Geometry check sheet. Reference: the model listing, model coordinates, mm. A direction names the side the tool comes from. Round coordinates to 2 decimals unless told otherwise and drop trailing zeros. Order: outer loops, then holes, each group sorted by start corner. A loop starts at its lowest first (then second) coordinate and runs counter-clockwise, first axis right, second up.
```python
from build123d import *

# Parameters (mm, degrees)
SKETCH1_R           = 1.5
BOSS_EXTRUDE1_DEPTH = 3
SKETCH4_R           = 1.5
CUT_EXTRUDE2_DEPTH  = 7
SKETCH5_W           = 46.5
SKETCH5_H           = 2
CUT_EXTRUDE3_DEPTH  = 7
CUT_EXTRUDE4_DEPTH  = 7
CUT_EXTRUDE5_DEPTH  = 7
BOSS_EXTRUDE2_START = -6
SKETCH8_R           = 1.5
BOSS_EXTRUDE2_DEPTH = 6
SKETCH9_R           = 1.5
CUT_EXTRUDE6_DEPTH  = 6
SKETCH10_R          = 1.5
CUT_EXTRUDE7_DEPTH  = 6
SKETCH11_W          = 36.769244088
SKETCH11_H          = 16.925373541
CUT_EXTRUDE8_DEPTH  = 14
FILLET2_R           = 5
FILLET3_R           = 10
FILLET4_R           = 20
FILLET5_R           = 30
FILLET6_R           = 10


with BuildPart() as part:
    # Sketch1 → Boss-Extrude1 (new body)
    # profile 1 of 4: a face of its own
    with BuildSketch(Plane(origin=(0, 0, 0), x_dir=(1, 0, 0), z_dir=(0, 1, 0))):
        Polygon((5, 16.666723622), (5, 56.73), (-5, 56.73), (-5, 5.234024539), (5, 5.234024539), (31.5, 5.234024539), (41.5, 5.234024539), (41.5, 64.6), (31.5, 64.6), (31.5, 54.48), (31.5, 16.666723622), align=None)
        with Locations(Location((0, 10.18, 0), (0, 0, 270))):
            Circle(SKETCH1_R, mode=Mode.SUBTRACT)
        with Locations(Location((36.5, 11.18, 0), (0, 0, 270))):
            Circle(SKETCH1_R, mode=Mode.SUBTRACT)
        with Locations(Location((0, 51.73, 0), (0, 0, 270))):
            Circle(SKETCH1_R, mode=Mode.SUBTRACT)
        with Locations(Location((36.5, 49.6, 0), (0, 0, 270))):
            Circle(SKETCH1_R, mode=Mode.SUBTRACT)
        with Locations(Location((36.5, 59.6, 0), (0, 0, 270))):
            Circle(SKETCH1_R, mode=Mode.SUBTRACT)
    # profile 2 of 4: a face of its own
    with BuildSketch(Plane(origin=(0, 0, 0), x_dir=(1, 0, 0), z_dir=(0, 1, 0))):
        Polygon((-5, 56.73), (5, 56.73), (31.5, 54.48), (31.5, 64.6), align=None)
    # profile 3 of 4: a face of its own
    with BuildSketch(Plane(origin=(0, 0, 0), x_dir=(1, 0, 0), z_dir=(0, 1, 0))):
        Polygon((5, 16.666723622), (5, 56.73), (-5, 56.73), (-5, 5.234024539), (5, 5.234024539), (31.5, 5.234024539), (41.5, 5.234024539), (41.5, 64.6), (31.5, 64.6), (31.5, 54.48), (31.5, 16.666723622), align=None)
        with Locations(Location((0, 10.18, 0), (0, 0, 270))):
            Circle(SKETCH1_R, mode=Mode.SUBTRACT)
        with Locations(Location((36.5, 11.18, 0), (0, 0, 270))):
            Circle(SKETCH1_R, mode=Mode.SUBTRACT)
        with Locations(Location((0, 51.73, 0), (0, 0, 270))):
            Circle(SKETCH1_R, mode=Mode.SUBTRACT)
        with Locations(Location((36.5, 49.6, 0), (0, 0, 270))):
            Circle(SKETCH1_R, mode=Mode.SUBTRACT)
        with Locations(Location((36.5, 59.6, 0), (0, 0, 270))):
            Circle(SKETCH1_R, mode=Mode.SUBTRACT)
    # profile 4 of 4: a face of its own
    with BuildSketch(Plane(origin=(0, 0, 0), x_dir=(1, 0, 0), z_dir=(0, 1, 0))):
        Polygon((31.5, 54.48), (5, 56.73), (5, 16.666723622), (31.5, 16.666723622), align=None)
    extrude(amount=BOSS_EXTRUDE1_DEPTH)

    # Sketch4 → Cut-Extrude2 (cut)
    with BuildSketch(Plane(origin=(0, 3, 0), x_dir=(1, 0, 0), z_dir=(0, 1, 0))):
        with Locations(Location((10, 51.73, 0), (0, 0, 270))):
            Circle(SKETCH4_R)
    extrude(amount=-CUT_EXTRUDE2_DEPTH, mode=Mode.SUBTRACT)

    # Sketch5 → Cut-Extrude3 (cut)
    with BuildSketch(Plane(origin=(0, 3, 0), x_dir=(1, 0, 0), z_dir=(0, 1, 0))):
        with Locations((18.25, 6.234024539)):
            Rectangle(SKETCH5_W, SKETCH5_H)
    extrude(amount=-CUT_EXTRUDE3_DEPTH, mode=Mode.SUBTRACT)

    # Sketch6 → Cut-Extrude4 (cut)
    with BuildSketch(Plane(origin=(0, 3, 0), x_dir=(1, 0, 0), z_dir=(0, 1, 0))):
        Polygon((31.443621834, 7.234024539), (-5, 42.312799573), (-5, 7.234024539), align=None)
    extrude(amount=-CUT_EXTRUDE4_DEPTH, mode=Mode.SUBTRACT)

    # Sketch7 → Cut-Extrude5 (cut)
    with BuildSketch(Plane(origin=(0, 3, 0), x_dir=(1, 0, 0), z_dir=(0, 1, 0))):
        Polygon((31.193110027, 22.772878628), (31.193110027, 44.066382221), (4.388346681, 44.066382221), align=None)
    extrude(amount=-CUT_EXTRUDE5_DEPTH, mode=Mode.SUBTRACT)

    # Sketch8 → Boss-Extrude2 (add)
    # profile 1 of 3: a face of its own
    with BuildSketch(Plane(origin=(0, 3, 0), x_dir=(1, 0, 0), z_dir=(0, 1, 0)).offset(BOSS_EXTRUDE2_START)):
        Polygon((238, 64.6), (41.5, 64.6), (41.5, 35.917012269), (208.144634928, 35.917012269), (201.5, 42.312799573), (201.5, 56.73), align=None)
    # profile 2 of 3: a face of its own
    with BuildSketch(Plane(origin=(0, 3, 0), x_dir=(1, 0, 0), z_dir=(0, 1, 0)).offset(BOSS_EXTRUDE2_START)):
        Polygon((237.943621834, 7.234024539), (248, 7.234024539), (248, 64.6), (238, 64.6), (201.5, 56.73), (201.5, 42.312799573), align=None)
        with Locations(Location((243, 11.18, 0), (0, 0, 270))):
            Circle(SKETCH8_R, mode=Mode.SUBTRACT)
        with Locations(Location((243, 59.6, 0), (0, 0, 270))):
            Circle(SKETCH8_R, mode=Mode.SUBTRACT)
        with Locations(Location((243, 49.6, 0), (0, 0, 270))):
            Circle(SKETCH8_R, mode=Mode.SUBTRACT)
        with Locations(Location((216.5, 51.73, 0), (0, 0, 270))):
            Circle(SKETCH8_R, mode=Mode.SUBTRACT)
        with Locations(Location((206.5, 51.73, 0), (0, 0, 270))):
            Circle(SKETCH8_R, mode=Mode.SUBTRACT)
        Polygon((237.693110027, 44.066382221), (237.693110027, 22.772878628), (210.888346681, 44.066382221), align=None, mode=Mode.SUBTRACT)
    # profile 3 of 3: a face of its own
    with BuildSketch(Plane(origin=(0, 3, 0), x_dir=(1, 0, 0), z_dir=(0, 1, 0)).offset(BOSS_EXTRUDE2_START)):
        Polygon((41.5, 35.917012269), (41.5, 64.6), (31.5, 64.6), (-5, 56.73), (-5, 42.312799573), (31.443621834, 7.234024539), (41.5, 7.234024539), align=None)
        with Locations(Location((36.5, 11.18, 0), (0, 0, 270))):
            Circle(SKETCH8_R, mode=Mode.SUBTRACT)
        Polygon((31.193110027, 22.772878628), (4.388346681, 44.066382221), (31.193110027, 44.066382221), align=None, mode=Mode.SUBTRACT)
        with Locations(Location((36.5, 49.6, 0), (0, 0, 270))):
            Circle(SKETCH8_R, mode=Mode.SUBTRACT)
        with Locations(Location((0, 51.73, 0), (0, 0, 270))):
            Circle(SKETCH8_R, mode=Mode.SUBTRACT)
        with Locations(Location((10, 51.73, 0), (0, 0, 270))):
            Circle(SKETCH8_R, mode=Mode.SUBTRACT)
        with Locations(Location((36.5, 59.6, 0), (0, 0, 270))):
            Circle(SKETCH8_R, mode=Mode.SUBTRACT)
    extrude(amount=BOSS_EXTRUDE2_DEPTH)

    # Sketch9 → Cut-Extrude6 (cut)
    with BuildSketch(Plane(origin=(0, 3, 0), x_dir=(1, 0, 0), z_dir=(0, 1, 0))):
        with Locations(Location((59.822317464, 50.258506135, 0), (0, 0, 270))):
            Circle(SKETCH9_R)
        with Locations(Location((189.822317464, 50.258506135, 0), (0, 0, 90))):
            Circle(SKETCH9_R)
        with Locations(Location((124.822317464, 50.258506135, 0), (0, 0, 270))):
            Circle(SKETCH9_R)
    extrude(amount=-CUT_EXTRUDE6_DEPTH, mode=Mode.SUBTRACT)

    # Sketch10 → Cut-Extrude7 (cut)
    with BuildSketch(Plane(origin=(0, 3, 0), x_dir=(1, 0, 0), z_dir=(0, 1, 0))):
        with Locations(Location((124.822317464, 50.258506135, 0), (0, 0, 270))):
            Circle(SKETCH10_R)
        with Locations(Location((109.822317464, 50.258506135, 0), (0, 0, 270))):
            Circle(SKETCH10_R)
        with Locations(Location((139.822317464, 50.258506135, 0), (0, 0, 270))):
            Circle(SKETCH10_R)
    extrude(amount=-CUT_EXTRUDE7_DEPTH, mode=Mode.SUBTRACT)

    # Sketch11 → Cut-Extrude8 (cut)
    with BuildSketch(Plane(origin=(0, 3, 0), x_dir=(1, 0, 0), z_dir=(0, 1, 0))):
        with Locations((84.822317464, 50.258506135)):
            Rectangle(SKETCH11_W, SKETCH11_H)
        with Locations((164.822317464, 50.258506135)):
            Rectangle(SKETCH11_W, SKETCH11_H)
    extrude(amount=-CUT_EXTRUDE8_DEPTH, mode=Mode.SUBTRACT)

    # Fillet2
    fillet2_edges = [part.edges().sort_by_distance(p)[0] for p in [
        (237.693110027, 0, -22.772878628),
        (237.693110027, 0, -44.066382221),
        (210.888346681, 0, -44.066382221),
        (31.193110027, 0, -22.772878628),
        (4.388346681, 0, -44.066382221),
        (31.193110027, 0, -44.066382221),
    ]]
    fillet(fillet2_edges, radius=FILLET2_R)

    # Fillet3
    # the kernel refuses this fillet: 10 mm, written as the material it adds along each edge
    with BuildSketch(Plane(origin=(183.206939508, 3, -41.795819364), x_dir=(-1, 0, 0), z_dir=(0, -1, 0)), Plane(origin=(146.43769542, 3, -41.795819364), x_dir=(0, 0, -1), z_dir=(0, -1, 0)), Plane(origin=(146.43769542, 3, -58.721192905), x_dir=(1, 0, 0), z_dir=(0, -1, 0)), Plane(origin=(103.206939508, 3, -41.795819364), x_dir=(-1, 0, 0), z_dir=(0, -1, 0)), Plane(origin=(66.43769542, 3, -58.721192905), x_dir=(1, 0, 0), z_dir=(0, -1, 0)), Plane(origin=(103.206939508, 3, -58.721192905), x_dir=(0, 0, 1), z_dir=(0, -1, 0))) as fillet3_piece_1:
        with BuildLine():
            CenterArc((FILLET3_R, FILLET3_R), FILLET3_R, 180, 90)
            Line((0, FILLET3_R), (0, 0))
            Line((0, 0), (FILLET3_R, 0))
        make_face()
    extrude(amount=6)
    with BuildSketch(Plane(origin=(183.206939508, 3, -58.721192905), x_dir=(-1, 0, 0), z_dir=(0, -1, 0)), Plane(origin=(66.43769542, 3, -41.795819364), x_dir=(1, 0, 0), z_dir=(0, -1, 0))) as fillet3_piece_2:
        with BuildLine():
            CenterArc((FILLET3_R, -FILLET3_R), FILLET3_R, 90, 90)
            Line((0, -FILLET3_R), (0, 0))
            Line((0, 0), (FILLET3_R, 0))
        make_face()
    extrude(amount=6)

    # Fillet4
    fillet4_edges = [part.edges().sort_by_distance(p)[0] for p in [
        (41.5, 0, -35.917012269),
    ]]
    fillet(fillet4_edges, radius=FILLET4_R)

    # Fillet5
    fillet5_edges = [part.edges().sort_by_distance(p)[0] for p in [
        (208.144634928, 0, -35.917012269),
    ]]
    fillet(fillet5_edges, radius=FILLET5_R)

    # Fillet6
    fillet6_edges = [part.edges().sort_by_distance(p)[0] for p in [
        (31.5, 0, -64.6),
    ]]
    fillet(fillet6_edges, radius=FILLET6_R)


solid = part.part
```
(1) Sectioned sample at B-B, the plane z = -23. Record the cut outline in (x, y).
Returned:
outline: (15.06, -3) - (42.8, -3) - (42.8, 3) - (15.06, 3) - close; (221.56, -3) - (248, -3) - (248, 3) - (221.56, 3) - close
(2) Draft check along Z on faces 1 (the cylindrical face through (29.77, -0.04, -42.56)), 2 (the flat face through (-5, 0, -50)), 3 (the flat face through (12.977, -0.042, -60.606)). Enter one of: released by +Z, released by -Z, zero draft, split by the parting line, or undercut.
Returned:
face 1: undercut
face 2: zero draft
face 3: released by -Z
(3) Depth check by flat-ended pin: P1, Ø1, axis at x = 124, y = 1.5, coming from the +Z side; P2, Ø3.5, axis at x = 243, z = -59.6, coming from the +Y side; P3, Ø1.8, axis at x = 36.5, z = -49.6, coming from the +Y side; P4, Ø3, axis at y = -1, z = -37, coming from the -X side. Enter the tip coordinate at first touch or a pass-through.
Returned:
P1: stops at z = -35.92
P2: stops at y = 3
P3: passes through
P4: stops at x = -1.04
(4) Material ranges on line 1 (Z direction, x = 243, y = 0.65); line 2 (Z direction, x = 83, y = 0.8); line 3 (X direction, y = 0.1, z = -45.5), recorded low to high.
Returned:
line 1: z = -64.6 to -61.1, -58.1 to -51.1, -48.1 to -12.68, -9.68 to -7.23
line 2: z = -64.6 to -58.72, -41.8 to -35.92
line 3: x = -5 to 68.67, 100.98 to 148.67, 180.98 to 248
(5) Sectioned sample at A-A, the plane x = 88.5. Record the cut outline in (y, z), and give its area (3 significant figures).
Returned:
outline: (-3, -64.6) - (3, -64.6) - (3, -58.72) - (-3, -58.72) - close; (-3, -41.8) - (3, -41.8) - (3, -35.92) - (-3, -35.92) - close
area: 70.5 mm2
(6) Set-up check for faces 4 (the cylindrical face through (149.858, 0.042, -56.251)), 5 (the flat face through (120, 3, -43)), 6 (the flat face through (41.5, 0, -12)): record each of +Z, -Z, +X, -X, +Y, -Y from which the full face is reachable in a straight line by a thin tool's end or side.
Returned:
face 4: +Y, -Y
face 5: +Z, -Z, +X, -X, +Y
face 6: +Z, +Y, -Y
(7) Sectioned sample at C-C, the plane y = -1.9. Give the number of separate pieces and of enclosed holes in the cut face, and give its area (3 significant figures).
Returned:
separate pieces: 1
enclosed holes: 19
area: 7,020 mm2
(8) Sectioned sample at D-D, the plane x = 49. Record the cut outline in (y, z).
Returned:
outline: (-3, -64.6) - (3, -64.6) - (3, -31.53) - (-3, -31.53) - close
